Autodesk Inventor part; units mm, degrees
ref_plane "YZ Plane" through (0, 0, 0) normal (1, 0, 0) x (0, 1, 0)
ref_plane "XZ Plane" through (0, 0, 0) normal (0, 1, 0) x (-1, 0, 0)
ref_plane "XY Plane" through (0, 0, 0) normal (0, 0, 1) x (1, 0, 0)
sketch "Sketch1" plane through (0, 0, 0) normal (0, 1, 0) x (-1, 0, 0)
  point P0 (0, 0)
sketch "Sketch2" plane through (0, 0, 0) normal (0, 1, 0) x (-1, 0, 0)
  line L0 (14, 10) -> (-14, 10)
  line L1 (-14, 10) -> (-14, -10)
  line L2 (-14, -10) -> (14, -10)
  line L3 (14, -10) -> (14, 10)
  point P0 (0, 0)
  dimension "d0" = 28
  dimension "d1" = 20
extrude "Extrusion1" add sketch "Sketch2" along normal blind 5
sketch "Sketch3" plane through (0, 5, 0) normal (0, 1, 0) x (1, 0, 0)
  circle A0 centre (7, 0) radius 2
  circle A1 centre (-7, 0) radius 2
  point P0 (0, 0)
  dimension "d4" = 4
  dimension "d5" = 4
extrude "Extrusion2" cut sketch "Sketch3" against normal blind 6
sketch "Sketch4" plane through (0, 5, 0) normal (0, 1, 0) x (1, 0, 0)
  line L0 (9.5, 4.5) -> (16.3647, 4.5)
  line L1 (16.3647, 4.5) -> (16.3647, 12.8099)
  line L2 (16.3647, 12.8099) -> (9.5, 12.8099)
  line L3 (9.5, 12.8099) -> (9.5, 4.5)
  point P0 (0, 0)
extrude "Extrusion3" cut sketch "Sketch4" against normal blind 6
chamfer "Chamfer1" distance 2 angle 45 5 edges at (-14, 2.5, -10) (9.5, 2.5, -10) (14, 2.5, -4.5) (14, 2.5, 10) (-14, 2.5, 10)
properties part number "gantryBeltCnctr"
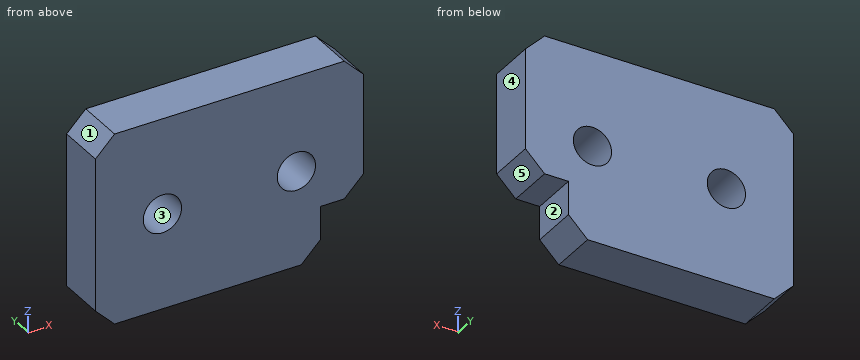
Check sheet for the modelled part. Datum: model origin and axes. Units: mm. Face numbers are marked on the shaded views. A direction names the side the tool comes from. Round coordinates to 2 decimals unless told otherwise and drop trailing zeros. Order: outer loops, then holes, each group sorted by start corner. A loop starts at its lowest first (then second) coordinate and runs counter-clockwise, first axis right, second up. Notation, with made-up numbers: M 72.25,83 L 79.25,83 A9 cw 79.25,88 Z; hole C 29,56.5 d4. An arc over 180 degrees is marked long. One line per item, written item: value. Start each with the question number.
1. Gauge pin test, flat ends, axial feed: P1, Ø6, axis at x = -5.5, z = 2.5, coming from the -Y side; P2, Ø1.2, axis at x = 10.5, y = 1.5, coming from the -Z side; P3, Ø1, axis at y = 3, z = -6, coming from the +X side. Record the tip position at first contact, or that the pin passes through.
2. Section check C-C on y = 0.8. Enter the section's corners in (x, z), and give its area (3 significant figures).
3. Scan lines: line 1 along X through (y, z) = (2, 0); line 2 along Z through (x, y) = (7, 2.9); line 3 along X through (y, z) = (3.65, -6.25). Record each from-to range of solid material in increasing order.
4. Section check B-B on z = 0. Enter the section's corners in (x, y), and give its area (3 significant figures).
5. Section check A-A on x = 7. Enter the section's corners in (y, z), and give its area (3 significant figures).
6. Release check for a two-part mould opening along Z. For the marked faces 3, 4 and 5 record: released by +Z, released by -Z, zero draft, split by the parting line, or undercut.
7. Access from +Z, -Z, +X, -X, +Y, -Y to the whole of each face (thin tool, end or side, straight path). Record for the marked faces 1 and 2.
8. Section check D-D on z = -8.5. Enter the section's corners in (x, y), and give its area (4 significant figures).
Results found:
1. P1: y = 0
1. P2: z = -4.5
1. P3: x = 9.5
2. outline: M -14,-8 L -12,-10 L 7.5,-10 L 9.5,-8 L 9.5,-4.5 L 12,-4.5 L 14,-2.5 L 14,8 L 12,10 L -12,10 L -14,8 Z; hole C -7,0 d4; hole C 7,0 d4
2. area: 500 mm^2
3. line 1: -14 to -9, -5 to 5, 9 to 14
3. line 2: -10 to -2, 2 to 10
3. line 3: -14 to 9.5
4. outline: M -14,0 L -9,0 L -9,5 L -14,5 Z; M -5,0 L 5,0 L 5,5 L -5,5 Z; M 9,0 L 14,0 L 14,5 L 9,5 Z
4. area: 100 mm^2
5. outline: M 0,-10 L 5,-10 L 5,-2 L 0,-2 Z; M 0,2 L 5,2 L 5,10 L 0,10 Z
5. area: 80.0 mm^2
6. face 3: undercut
6. face 4: zero draft
6. face 5: released by -Z
7. face 1: +Z, -X, +Y, -Y
7. face 2: -Z, +X, +Y, -Y
8. outline: M -13.5,0 L 9,0 L 9,5 L -13.5,5 Z
8. area: 112.5 mm^2
